from build123d import *

# Parameters (mm, degrees)
SKETCH1_R           = 1.5
SKETCH1_W           = 20
SKETCH1_H           = 5
BOSS_EXTRUDE3_DEPTH = 3
FILLET2_R           = 5
CUT_EXTRUDE1_REACH  = 74.753
SKETCH3_W           = 28.786192162
SKETCH3_H           = 21.000620262
FILLET3_R           = 5
SKETCH5_W           = 10
SKETCH5_H           = 10
CUT_EXTRUDE2_DEPTH  = 10
BOSS_EXTRUDE5_START = -3
SKETCH8_W           = 35
SKETCH8_H           = 15
SKETCH8_R           = 1.5
BOSS_EXTRUDE5_DEPTH = 3
CUT_EXTRUDE3_REACH  = 62.523
SKETCH9_W           = 10
SKETCH9_H           = 10
SKETCH9_W_2         = 11
FILLET4_R           = 5


with BuildPart() as part:
    # Sketch1 → Boss-Extrude3 (new body)
    # profile 1 of 3: a face of its own
    with BuildSketch(Plane(origin=(0, 0, 0), x_dir=(1, 0, 0), z_dir=(0, 1, 0))):
        Polygon((10, 55), (-10, 55), (-10, -30), (-7, -30), (-7, -34.5), (-10, -34.5), (-10, -50), (10, -50), (10, -34.5), (7, -34.5), (7, -30), (10, -30), align=None)
        with Locations(Location((-5, -48, 0), (0, 0, 270))):
            Circle(SKETCH1_R, mode=Mode.SUBTRACT)
        with Locations(Location((-5, 2, 0), (0, 0, 270))):
            Circle(SKETCH1_R, mode=Mode.SUBTRACT)
        with Locations(Location((-5, 52, 0), (0, 0, 270))):
            Circle(SKETCH1_R, mode=Mode.SUBTRACT)
    # profile 2 of 3: a face of its own
    with BuildSketch(Plane(origin=(0, 0, 0), x_dir=(1, 0, 0), z_dir=(0, 1, 0))):
        Polygon((10, -55), (-10, -55), (-10, -64.5), (-7, -64.5), (-7, -69), (-10, -69), (-10, -72), (10, -72), (10, -69), (7, -69), (7, -64.5), (10, -64.5), align=None)
    # profile 3 of 3: a face of its own
    with BuildSketch(Plane(origin=(0, 0, 0), x_dir=(1, 0, 0), z_dir=(0, 1, 0))):
        with Locations((0, -52.5)):
            Rectangle(SKETCH1_W, SKETCH1_H)
    extrude(amount=BOSS_EXTRUDE3_DEPTH)

    # Fillet2
    # the kernel refuses this fillet: 5 mm, written as the material it takes off along each edge
    with BuildSketch(Plane(origin=(10, -11.456439237, 72), x_dir=(0, 0, -1), z_dir=(0, 1, 0))) as fillet2_piece_1:
        with BuildLine():
            CenterArc((5, 4.582575695), FILLET2_R, 180, 66.421821522)
            Line((0, 4.582575695), (-0.1, 4.582575695))
            Line((-0.1, 4.582575695), (-0.1, 0))
            Line((-0.1, 0), (0, -0.1))
            ThreePointArc((0, -0.1), (1.5, -0.1), (2.96, -0.091651514))
            Line((2.96, -0.091651514), (3, 0))
        make_face()
    extrude(amount=25.912878475, mode=Mode.SUBTRACT)
    with BuildSketch(Plane(origin=(-10, -11.456439237, 72), x_dir=(1, 0, 0), z_dir=(0, 1, 0))) as fillet2_piece_2:
        with BuildLine():
            CenterArc((4.582575695, 5), FILLET2_R, 203.578178478, 66.421821522)
            Line((0, 3), (-0.091651514, 2.96))
            ThreePointArc((-0.091651514, 2.96), (-0.1, 1.5), (-0.1, 0))
            Line((-0.1, 0), (0, -0.1))
            Line((0, -0.1), (4.582575695, -0.1))
            Line((4.582575695, -0.1), (4.582575695, 0))
        make_face()
    extrude(amount=25.912878475, mode=Mode.SUBTRACT)
    with BuildSketch(Plane(origin=(-10, -12.5, -55), x_dir=(0, 0, 1), z_dir=(0, 1, 0))) as fillet2_piece_3:
        with BuildLine():
            CenterArc((FILLET2_R, FILLET2_R), FILLET2_R, 180, 90)
            Line((0, FILLET2_R), (-FILLET2_R * 0.02, FILLET2_R))
            Line((-FILLET2_R * 0.02, FILLET2_R), (-FILLET2_R * 0.02, -FILLET2_R * 0.02))
            Line((-FILLET2_R * 0.02, -FILLET2_R * 0.02), (FILLET2_R, -FILLET2_R * 0.02))
            Line((FILLET2_R, -FILLET2_R * 0.02), (FILLET2_R, 0))
        make_face()
    extrude(amount=28, mode=Mode.SUBTRACT)
    with BuildSketch(Plane(origin=(10, -12.5, -55), x_dir=(0, 0, 1), z_dir=(0, 1, 0))) as fillet2_piece_4:
        with BuildLine():
            CenterArc((FILLET2_R, -FILLET2_R), FILLET2_R, 90, 90)
            Line((0, -FILLET2_R), (-FILLET2_R * 0.02, -FILLET2_R))
            Line((-FILLET2_R * 0.02, -FILLET2_R), (-FILLET2_R * 0.02, FILLET2_R * 0.02))
            Line((-FILLET2_R * 0.02, FILLET2_R * 0.02), (FILLET2_R, FILLET2_R * 0.02))
            Line((FILLET2_R, FILLET2_R * 0.02), (FILLET2_R, 0))
        make_face()
    extrude(amount=28, mode=Mode.SUBTRACT)

    # Sketch3 → Cut-Extrude1 (cut, up to next)
    with BuildSketch(Plane(origin=(0, 3, 0), x_dir=(1, 0, 0), z_dir=(0, 1, 0)), mode=Mode.PRIVATE) as cut_extrude1_sk1:
        with Locations((0, -63.390803798)):
            Rectangle(SKETCH3_W, SKETCH3_H)
    cut_extrude1_tool1 = extrude(cut_extrude1_sk1.sketch, amount=-CUT_EXTRUDE1_REACH, mode=Mode.PRIVATE) & part.part
    add(cut_extrude1_tool1.solids().sort_by_distance((0, 3, 63.390804))[0], mode=Mode.SUBTRACT)

    # Fillet3
    fillet3_edges = [part.edges().sort_by_distance(p)[0] for p in [
        (10, 1.5, 52.890493667),
        (-10, 1.5, 52.890493667),
    ]]
    fillet(fillet3_edges, radius=FILLET3_R)

    # Sketch5 → Cut-Extrude2 (cut)
    with BuildSketch(Plane(origin=(0, 3, 0), x_dir=(1, 0, 0), z_dir=(0, 1, 0))):
        with Locations((0, -53)):
            Rectangle(SKETCH5_W, SKETCH5_H)
        with Locations((0, 47)):
            Rectangle(SKETCH5_W, SKETCH5_H)
    extrude(amount=-CUT_EXTRUDE2_DEPTH, mode=Mode.SUBTRACT)

    # Sketch8 → Boss-Extrude5 (add)
    with BuildSketch(Plane(origin=(0, 3, 0), x_dir=(1, 0, 0), z_dir=(0, 1, 0)).offset(BOSS_EXTRUDE5_START)):
        with Locations((7.580003557, -2.462217959)):
            Rectangle(SKETCH8_W, SKETCH8_H)
        with Locations(Location((15, 2, 0), (0, 0, 270))):
            Circle(SKETCH8_R, mode=Mode.SUBTRACT)
        with Locations(Location((-5, 2, 0), (0, 0, 270))):
            Circle(SKETCH8_R, mode=Mode.SUBTRACT)
    extrude(amount=BOSS_EXTRUDE5_DEPTH)

    # Sketch9 → Cut-Extrude3 (cut, up to next)
    with BuildSketch(Plane(origin=(0, 3, 0), x_dir=(1, 0, 0), z_dir=(0, 1, 0)), mode=Mode.PRIVATE) as cut_extrude3_sk1:
        with Locations((0, -3)):
            Rectangle(SKETCH9_W, SKETCH9_H)
    cut_extrude3_tool1 = extrude(cut_extrude3_sk1.sketch, amount=-CUT_EXTRUDE3_REACH, mode=Mode.PRIVATE) & part.part
    # Sketch9 → Cut-Extrude3 (cut, up to next)
    with BuildSketch(Plane(origin=(0, 3, 0), x_dir=(1, 0, 0), z_dir=(0, 1, 0)), mode=Mode.PRIVATE) as cut_extrude3_sk2:
        with Locations((20.5, -3)):
            Rectangle(SKETCH9_W_2, SKETCH9_H)
    cut_extrude3_tool2 = extrude(cut_extrude3_sk2.sketch, amount=-CUT_EXTRUDE3_REACH, mode=Mode.PRIVATE) & part.part
    add(cut_extrude3_tool1.solids().sort_by_distance((0, 3, 3))[0], mode=Mode.SUBTRACT)
    add(cut_extrude3_tool2.solids().sort_by_distance((20.5, 3, 3))[0], mode=Mode.SUBTRACT)

    # Fillet4
    # the kernel refuses this fillet: 5 mm, written as the material it adds along each edge
    with BuildSketch(Plane(origin=(10, 0, 9.962217959), x_dir=(1, 0, 0), z_dir=(0, 1, 0))) as fillet4_piece_1:
        with BuildLine():
            CenterArc((FILLET4_R, -FILLET4_R), FILLET4_R, 90, 90)
            Line((0, -FILLET4_R), (0, 0))
            Line((0, 0), (FILLET4_R, 0))
        make_face()
    extrude(amount=3)
    with BuildSketch(Plane(origin=(10, 3, -5.037782041), x_dir=(0, 0, -1), z_dir=(0, -1, 0))) as fillet4_piece_2:
        with BuildLine():
            CenterArc((FILLET4_R, FILLET4_R), FILLET4_R, 180, 90)
            Line((0, FILLET4_R), (0, 0))
            Line((0, 0), (FILLET4_R, 0))
        make_face()
    extrude(amount=3)
    # the kernel refuses this fillet: 5 mm, written as the material it takes off along each edge
    with BuildSketch(Plane(origin=(25.080003557, -9.928456662, 9.962217959), x_dir=(0, 0, -1), z_dir=(0, 1, 0))) as fillet4_2_piece_1:
        with BuildLine():
            CenterArc((5, 3.971382665), FILLET4_R, 180, 52.586975679)
            Line((0, 3.971382665), (0, 0))
            Line((0, 0), (1.962217959, 0))
        make_face()
    extrude(amount=22.856913325, mode=Mode.SUBTRACT)
    with BuildSketch(Plane(origin=(25.080003557, -11.497200931, -5.037782041), x_dir=(-1, 0, 0), z_dir=(0, 1, 0))) as fillet4_2_piece_2:
        with BuildLine():
            CenterArc((4.598880373, 5), FILLET4_R, 203.106632515, 66.893367485)
            Line((0, 3.037782041), (0, 0))
            Line((0, 0), (4.598880373, 0))
        make_face()
    extrude(amount=25.994401863, mode=Mode.SUBTRACT)


solid = part.part
The model under review builds one solid part; all positions refer to its coordinate system, in mm. A direction names the side the tool comes from. Round coordinates to 2 decimals unless told otherwise and drop trailing zeros. Loops run counter-clockwise (first coordinate to the right, second up) from the corner with the lowest first, then second, coordinate; pieces in that order, holes last. Notation, with made-up numbers: (46.25, 46) - (71.25, 46) arc R38 cw to (71.25, 85) - close; hole circle Ø11 at (61.5, -7.5). An arc over 180 degrees is marked (long way). Use CSV: the item, a comma, the result in double quotes.
(1) Take a section at A-A, the plane z = -44.5. Give the boundary of the cut face in (x, y).
Working result:
outline,"(-10, 0) - (-5, 0) - (-5, 3) - (-10, 3) - close; (5, 0) - (10, 0) - (10, 3) - (5, 3) - close"
(2) Machinability: for faces 4 (the flat face through (9, 1, 34.5)), 5 (the flat face through (10, 1, 23)), 6 (the flat face through (5, 2, -47)), 7 (the flat face through (-10, 1, 41)), 8 (the cylindrical face through (9, 1, -53)), which of the approach directions +Z, -Z, +X, -X, +Y, -Y give a long, thin tool a straight path to every point of the face, cutting with its end or side? Answer none if there is none.
Working result:
face 4,"+X, +Y, -Y"
face 5,"+Z, +X, +Y, -Y"
face 6,"+Y, -Y"
face 7,"+Z, -Z, -X, +Y, -Y"
face 8,"-Z, +X, +Y, -Y"
(3) Clearance check with flat-ended pins moving along their axes: P1, Ø0.9, axis at x = 17, y = 2, coming from the +Z side; P2, Ø5, axis at x = 13, z = 31.5, coming from the -Y side; P3, Ø1.5, axis at y = 2, z = 21.5, coming from the +X side; P4, Ø1.5, axis at y = 1, z = 49.5, coming from the -X side. State where each tip first meets the part, or that it passes through.
Working result:
P1,"stops at z = 9.96"
P2,"passes through"
P3,"stops at x = 10"
P4,"stops at x = -9.93"
(4) Take a section at B-B, the plane x = -8. Give the boundary of the cut face in (y, z), plus the area to 3 significant figures.
Working result:
outline,"(0, -54) - (3, -54) - (3, 30) - (0, 30) - close; (0, 34.5) - (3, 34.5) - (3, 51.89) - (0, 51.89) - close"
area,"304 mm^2"
(5) The part is to be moulded in two halves that separate along Z. For faces 1 (the flat face through (8, 0, -2)), 2 (the flat face through (18, 1, -5.038)), 3 (the flat face through (-9, 1, 30)), say which applies: pulls with the +Z half, pulls with the -Z half, needs draft (parallel to the pull), parting line crosses it, or undercut.
Working result:
face 1,"needs draft"
face 2,"pulls with the -Z half"
face 3,"undercut"
(6) Take a section at D-D, the plane z = 25.5. Give the boundary of the cut face in (x, y), plus the area to 3 significant figures.
Working result:
outline,"(-10, 0) - (10, 0) - (10, 3) - (-10, 3) - close"
area,"60.0 mm^2"
(7) Take a section at C-C, the plane y = 1.15. State how many separate pieces and enclosed holes the cut face has, plus the area to 3 significant figures.
Working result:
separate pieces,"1"
enclosed holes,"2"
area,"1,970 mm^2"
(8) For line 1 (Z direction, x = 0, y = 1.25); line 2 (Z direction, x = -6, y = 2.3); line 3 (X direction, y = 0.9, z = 1.5), list the stretches that pass through material, from the lowest coordinate up.
Working result:
line 1,"z = -55 to -52, -42 to -2, 8 to 48"
line 2,"z = -54.9 to -53.12, -50.88 to -3.12, -0.88 to 46.88, 49.12 to 52.79"
line 3,"x = -10 to -5, 5 to 15"
